Geometry check sheet. Reference: the model listing, model coordinates, mm. A direction names the side the tool comes from. Give positions to 0.01 mm unless a question says otherwise; leave off trailing zeros. Loops run counter-clockwise (first coordinate to the right, second up) from the corner with the lowest first, then second, coordinate; pieces in that order, holes last. Notation, with made-up numbers: (71, 79.25) -> (93, 79.25) arc R21 cw to (93, 83.25) -> close; hole circle Ø9 at (16, 22). An arc over 180 degrees is marked (long way). Write item = value, one per line.
```python
from build123d import *

# Parameters (mm, degrees)
SKETCH1_W           = 25.4
SKETCH1_H           = 25.4
SKETCH1_W_2         = 22.225
SKETCH1_H_2         = 22.225
BOSS_EXTRUDE1_DEPTH = 431.8
SKETCH2_R           = 3.175
CUT_EXTRUDE1_DEPTH  = 26.4
CUT_EXTRUDE2_DEPTH  = 491.49


with BuildPart() as part:
    # Sketch1 → Boss-Extrude1 (new body)
    with BuildSketch(Plane.XY):
        Rectangle(SKETCH1_W, SKETCH1_H)
        Rectangle(SKETCH1_W_2, SKETCH1_H_2, mode=Mode.SUBTRACT)
    extrude(amount=BOSS_EXTRUDE1_DEPTH)

    # Sketch2 → Cut-Extrude1 (cut, through all)
    with BuildSketch(Plane(origin=(12.7, 0, 0), x_dir=(0, 0, -1), z_dir=(1, 0, 0))):
        with Locations((-419.1, 0)):
            Circle(SKETCH2_R)
        with Locations((-7.62, 0)):
            Circle(SKETCH2_R)
        with Locations((-20.32, 0)):
            Circle(SKETCH2_R)
    extrude(amount=-CUT_EXTRUDE1_DEPTH, mode=Mode.SUBTRACT)

    # Sketch4 → Cut-Extrude2 (cut)
    with BuildSketch(Plane(origin=(12.7, 0, 0), x_dir=(0, 0, -1), z_dir=(1, 0, 0))):
        with BuildLine():
            Line((-419.1, 12.7), (-431.8, 12.7))
            Line((-431.8, 12.7), (-491.49, -12.7))
            Line((-491.49, -12.7), (-419.1, -12.7))
            ThreePointArc((-419.1, -12.7), (-431.8, 0), (-419.1, 12.7))
        make_face()
    extrude(amount=-CUT_EXTRUDE2_DEPTH, mode=Mode.SUBTRACT)


solid = part.part
```
Item 1: Section check B-B, the plane x = -4.5. Record the cut outline in (y, z).
Answer:
outline = (-12.7, 0) -> (-11.11, 0) -> (-11.11, 425.25) arc R12.7 ccw to (-12.7, 419.1) -> close; (11.11, 0) -> (12.7, 0) -> (12.7, 419.1) arc R12.7 ccw to (11.11, 425.25) -> close
Item 2: Section check A-A, the plane z = 336.5. Record the cut outline in (x, y), plus the area to 3 significant figures.
Answer:
outline = (-12.7, -12.7) -> (12.7, -12.7) -> (12.7, 12.7) -> (-12.7, 12.7) -> close; hole (-11.11, -11.11) -> (11.11, -11.11) -> (11.11, 11.11) -> (-11.11, 11.11) -> close
area = 151 mm^2
Item 3: Draft check along Y on faces 3 (the cylindrical face through (3, -12.553, 421.03)), 4 (the flat face through (0, 12.7, 207)), 5 (the flat face through (0, -11.112, 210)), 6 (the flat face through (11.112, 0, 213)). Enter one of: +Y half, -Y half, draft (parallel to the pull), parting line (faces both ways), or undercut.
Answer:
face_3 = parting line
face_4 = +Y half
face_5 = undercut
face_6 = undercut
Item 4: Tool access check on faces 1 (the flat face through (12.7, 0, 213)), 2 (the flat face through (-11.112, 0, 213)). Record the directions out of +Z, -Z, +X, -X, +Y, -Y that give a thin tool (end or side, any length) a straight path to the whole face; none if there is none.
Answer:
face_1 = +Z, -Z, +X, +Y, -Y
face_2 = +Z, -Z
Item 5: Thickness scan on L1, parallel to X at y = -3.5, z = 144.5; L2, parallel to Y at x = -11.7, z = 20.32 (3 decimals). Record the ranges inside material, lowest first. Write a range as [from, to].
Answer:
L1 = [-12.7, -11.11], [11.11, 12.7]
L2 = [-12.7, -3.175], [3.175, 12.7]
